Autodesk Inventor part; units mm, degrees
ref_plane "YZ Plane" through (0, 0, 0) normal (1, 0, 0) x (0, 1, 0)
ref_plane "XZ Plane" through (0, 0, 0) normal (0, 1, 0) x (-1, 0, 0)
ref_plane "XY Plane" through (0, 0, 0) normal (0, 0, 1) x (1, 0, 0)
sketch "Sketch1" plane through (0, 0, 0) normal (0, 1, 0) x (-1, 0, 0)
  line L0 (6.35, 26.2509) -> (-6.35, 26.2509)
  line L1 (-6.35, 26.2509) -> (-6.35, -26.2509)
  line L2 (-6.35, -26.2509) -> (6.35, -26.2509)
  line L3 (6.35, -26.2509) -> (6.35, 26.2509)
  point P0 (0, 0)
  dimension "d0" = 6.35
  dimension "d1" = 12.7
  dimension "d2" = 52.5018
  dimension "d3" = 26.2509
extrude "Extrusion1" add sketch "Sketch1" along normal blind 22.225
fillet "Fillet1" radius 3.175 1 edges at (6.35, 22.225, 0)
sketch "Sketch2" plane through (-6.35, 0, -26.2509) normal (-1, 0, 0) x (0, 0, 1)
  line L0 (52.5018, 19.05) -> (0, 19.05)
  line L1 (0, 0) -> (0, 22.225)
  line L2 (52.5018, 0) -> (52.5018, 22.225)
  line L3 (8.3439, 22.225) -> (9.6139, 22.225)
  line L4 (9.6139, 22.225) -> (9.6139, 20.447)
  line L5 (9.6139, 20.447) -> (8.3439, 20.447)
  line L6 (8.3439, 20.447) -> (8.3439, 22.225)
  line L7 (17.1069, 22.225) -> (18.1229, 22.225)
  line L8 (18.1229, 22.225) -> (18.1229, 20.447)
  line L9 (18.1229, 20.447) -> (17.1069, 20.447)
  line L10 (17.1069, 20.447) -> (17.1069, 22.225)
  line L11 (25.8699, 22.225) -> (26.6319, 22.225)
  line L12 (26.6319, 22.225) -> (26.6319, 20.447)
  line L13 (26.6319, 20.447) -> (25.8699, 20.447)
  line L14 (25.8699, 20.447) -> (25.8699, 22.225)
  line L15 (34.6075, 22.225) -> (35.1663, 22.225)
  line L16 (35.1663, 22.225) -> (35.1663, 20.447)
  line L17 (35.1663, 20.447) -> (34.6075, 20.447)
  line L18 (34.6075, 20.447) -> (34.6075, 22.225)
  line L19 (43.2689, 22.225) -> (43.7769, 22.225)
  line L20 (43.7769, 22.225) -> (43.7769, 20.447)
  line L21 (43.7769, 20.447) -> (43.2689, 20.447)
  line L22 (43.2689, 20.447) -> (43.2689, 22.225)
  line L23 (8.9789, 20.447) -> (17.6149, 20.447) construction
  line L24 (17.6149, 20.447) -> (26.2509, 20.447) construction
  line L25 (26.2509, 20.447) -> (34.8869, 20.447) construction
  line L26 (34.8869, 20.447) -> (43.5229, 20.447) construction
  arc A0 (8.3439, 20.447) -> (9.6139, 20.447) centre (8.9789, 20.447) ccw
  arc A1 (17.1069, 20.447) -> (18.1229, 20.447) centre (17.6149, 20.447) ccw
  arc A2 (25.8699, 20.447) -> (26.6319, 20.447) centre (26.2509, 20.447) ccw
  arc A3 (34.6075, 20.447) -> (35.1663, 20.447) centre (34.8869, 20.447) ccw
  arc A4 (43.2689, 20.447) -> (43.7769, 20.447) centre (43.5229, 20.447) ccw
  line L27 (34.6075, 22.225) -> (35.1663, 22.225)
  line L28 (43.2689, 22.225) -> (43.7769, 22.225)
  line L29 (25.8699, 22.225) -> (26.6319, 22.225)
  line L30 (8.3439, 22.225) -> (9.6139, 22.225)
  line L31 (17.1069, 22.225) -> (18.1229, 22.225)
  line L32 (0, 22.225) -> (52.5018, 22.225)
  line L33 (8.9789, 20.447) -> (0, 20.447) construction
  line L34 (43.5229, 20.447) -> (52.5018, 20.447) construction
  point P0 (26.2509, 0)
  dimension "d20" = 1.27
  dimension "d21" = 1.016
  dimension "d22" = 0.762
  dimension "d23" = 0.508
  dimension "d24" = 0.5588
  dimension "d25" = 1.778
  dimension "d26" = 8.636
extrude "Extrusion4" cut sketch "Sketch2" against normal blind 25.4 contours L20 L21 L22 L19 | L3 L4 L5 L6 | A4 L21 | L5 A0 | L16 L17 L18 L15 | L7 L8 L9 L10 | A3 L17 | L9 A1 | L12 L13 L14 L11 | A2 L13
properties part number "Nut0" material "LCP Plastic"
Geometry check sheet. Reference: the model listing, model coordinates, mm. A direction names the side the tool comes from. Coordinates: 2 decimals unless noted, no trailing zeros.
Item 1: Release check for a two-part mould opening along X. For faces 1 (the face through (-6.35, 11, 0)), 2 (the face through (6.23, 19.91, -0.37)), 3 (the face through (0, 21, -8.128)) record: released by +X, released by -X, zero draft, split by the parting line, or undercut.
Item 2: Access from +Z, -Z, +X, -X, +Y, -Y to the whole of each face (thin tool, end or side, straight path). Record for faces 4 (the face through (0, 21, -9.144)), 5 (the face through (-2, 22.225, -13)).
Item 3: Thickness scan on line 1 (Z direction, x = 3.25, y = 21.25); line 2 (Y direction, x = 5.75, z = 9.5); line 3 (X direction, y = 21.25, z = 7.5). Record the ranges inside material, lowest first.
Item 4: Go/stop test with a flat-tipped pin: pin 1 Ø1.5 at (x, z) = (4.5, 3) entering from +Y. Record where the tip stops, or that it passes through.
Check result:
1. face 1: released by -X
1. face 2: released by +X
1. face 3: zero draft
2. face 4: +X, -X, +Y
2. face 5: +Z, -Z, +X, -X, +Y
3. line 1: z = -26.25 to -17.91, -16.64 to -9.14, -8.13 to -0.38, 0.38 to 8.36, 8.92 to 17.02, 17.53 to 26.25
3. line 2: y = 0 to 20.91
3. line 3: x = -6.35 to 5.46
4. pin 1: stops at y = 22.17
